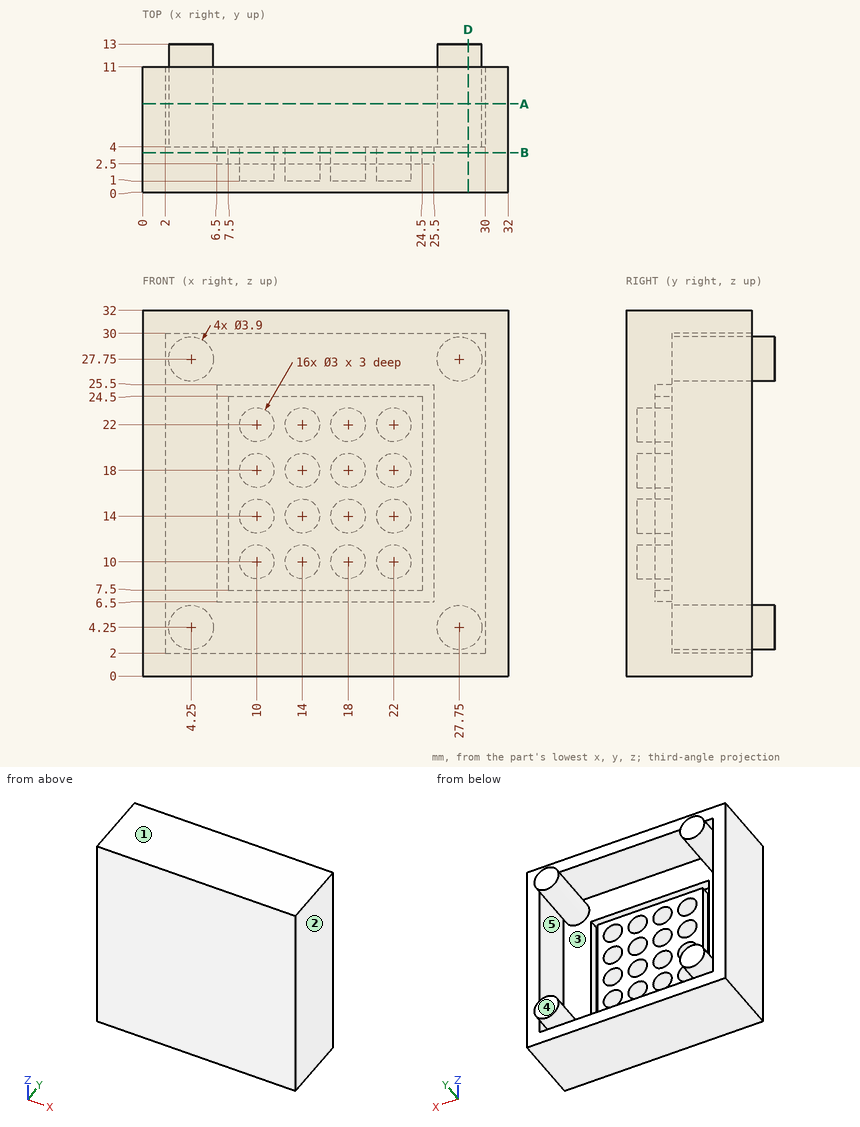
Here's the drawing with two shaded views (mm, measured from the low corner). I have some questions. A direction names the side the tool comes from. Round coordinates to 2 decimals unless told otherwise and drop trailing zeros. Loops run counter-clockwise (first coordinate to the right, second up) from the corner with the lowest first, then second, coordinate; pieces in that order, holes last.
Item 1: Suppose I cut it at D-D, the plane x = 28.5. Write out the boundary of the cut face in (y, z), then the cut area to 3 significant figures.
Item 2: Which directions (+Z, -Z, +X, -X, +Y, -Y) give clear straight access to the entire face, cutting with the end or side of a thin tool? Please do the marked faces 4 and 5.
Item 3: Will these pins go through, and if not, where does the flat tip stop? pin 1 Ø18.5 at (x, z) = (12.5, 12) entering from +Y; pin 2 Ø1.8 at (x, z) = (18, 18) entering from +Y.
Item 4: Suppose I cut it at A-A, the plane y = 7.75. Write out the boundary of the cut face in (x, z).
Item 5: Suppose I cut it at B-B, the plane y = 3.5. State how many separate pieces and enclosed holes the cut face has, then the cut area to 3 significant figures.
Item 6: If we mould it in two halves opening along X, with no side actions, what happens to the marked faces 1, 2 and 3? For each: +X half, -X half, draft (parallel to the pull), parting line (faces both ways), or undercut.
Item 7: Please list where these lines run through material, in increasing order: L1, parallel to Z at x = 18, y = 2.4; L2, parallel to X at y = 6.25, z = 14.5.
Reported:
1. outline: (0, 0) - (11, 0) - (11, 2) - (4, 2) - (4, 2.45) - (13, 2.45) - (13, 6.05) - (4, 6.05) - (4, 25.95) - (13, 25.95) - (13, 29.55) - (4, 29.55) - (4, 30) - (11, 30) - (11, 32) - (0, 32) - close
1. area: 221 mm2
2. face 4: +Z, -Z, +X, -X, +Y
2. face 5: +Y
3. pin 1: stops at y = 4
3. pin 2: stops at y = 1
4. outline: (0, 0) - (32, 0) - (32, 32) - (0, 32) - close; circle Ø3.9 at (4.25, 4.25); circle Ø3.9 at (4.25, 27.75); circle Ø3.9 at (27.75, 4.25); circle Ø3.9 at (27.75, 27.75); hole (2, 2) - (30, 2) - (30, 30) - (2, 30) - close
5. separate pieces: 2
5. enclosed holes: 17
5. area: 839 mm2
6. face 1: draft
6. face 2: +X half
6. face 3: undercut
7. L1: z = 0 to 8.5, 11.5 to 12.5, 15.5 to 16.5, 19.5 to 20.5, 23.5 to 32
7. L2: x = 0 to 2, 30 to 32
